The listing builds one solid part. Answer for the finished solid, in the listing's coordinates (mm). Face numbers are marked on the shaded views. A direction names the side the tool comes from. Round coordinates to 2 decimals unless told otherwise and drop trailing zeros. Loops run counter-clockwise (first coordinate to the right, second up) from the corner with the lowest first, then second, coordinate; pieces in that order, holes last. Notation, with made-up numbers: M 9,-17 L 44,-17 A31 ccw 44,9 Z; hole C -31.75,-27 d10. An arc over 180 degrees is marked long. Put each result on its own line as item: value. Start each with the question number.
(1) Straight lines are drawn through the part: line 1 (X direction, y = 12, z = 17.5); line 2 (X direction, y = 63, z = 2.25); line 3 (Z direction, x = 52, y = 34). For each, find the intervals that lie inside material, in ascending order.
(2) Determine the mould class of the marked faces 4, 5 and 6 for opening direction X: released by +X, released by -X, zero draft, split by the parting line, or undercut.
(3) Section A-A, the plane z = 22 is taken. Determine the outline of the cut face in (x, y).
(4) Section C-C, the plane x = 10 is taken. Determine the outline of the cut face in (y, z), then the cut area to 3 significant figures.
(5) Section B-B, the plane y = 14.5 is taken. Determine the outline of the cut face in (x, z), then the cut area to 3 significant figures.
(6) Flat-ended cylindrical pins translate along their axes: P1, Ø10, axis at x = 51, y = 19.5, coming from the -Z side; P2, Ø10.5, axis at y = 41.5, z = 10.5, coming from the +X side; P3, Ø21, axis at x = 71.5, y = 27, coming from the +Z side; P4, Ø6.5, axis at y = 34, z = 11.5, coming from the -X side. Find the tip coordinate at first contact, or state that the pin passes through.
(7) Which of the six approach directions +Z, -Z, +X, -X, +Y, -Y give full straight-line access (tool end or side, diameter ignored) to the marked faces 1, 2 and 3?
(8) Section D-D, the plane z = 2.75 is taken. Determine the outline of the cut face in (x, y), then the cut area to 3 significant figures.
```python
from build123d import *

# Parameters (mm, degrees)
SKETCH_1_W          = 120
SKETCH_1_H          = 75
EXTRUDE_1_DEPTH     = 4
SKETCH_2_W          = 5
SKETCH_2_H          = 75
EXTRUDE_2_DEPTH     = 21
CUT_EXTRUDE_1_DEPTH = 144.701078632


with BuildPart() as part:
    # 草图1 → 凸台-拉伸1 (new body)
    with BuildSketch(Plane.XY):
        with Locations((60, 37.5)):
            Rectangle(SKETCH_1_W, SKETCH_1_H)
    extrude(amount=EXTRUDE_1_DEPTH)

    # 草图2 → 凸台-拉伸2 (add)
    with BuildSketch(Plane.XY.offset(4)):
        with Locations((22.5, 37.5)):
            Rectangle(SKETCH_2_W, SKETCH_2_H)
        with Locations((97.5, 37.5)):
            Rectangle(SKETCH_2_W, SKETCH_2_H)
    extrude(amount=EXTRUDE_2_DEPTH)

    # 草图3 → 切除-拉伸1 (cut, through all)
    with BuildSketch(Plane(origin=(0, 0, 0), x_dir=(-1, 0, 0), z_dir=(0, 0, -1))):
        with BuildLine():
            Line((-112.5, 65), (-112.5, 55))
            ThreePointArc((-112.5, 55), (-110, 52.5), (-107.5, 55))
            Line((-107.5, 55), (-107.5, 65))
            ThreePointArc((-107.5, 65), (-110, 67.5), (-112.5, 65))
        make_face()
        with BuildLine():
            Line((-107.5, 10), (-107.5, 20))
            ThreePointArc((-107.5, 20), (-110, 22.5), (-112.5, 20))
            Line((-112.5, 20), (-112.5, 10))
            ThreePointArc((-112.5, 10), (-110, 7.5), (-107.5, 10))
        make_face()
        with BuildLine():
            Line((-7.5, 10), (-7.5, 20))
            ThreePointArc((-7.5, 20), (-10, 22.5), (-12.5, 20))
            Line((-12.5, 20), (-12.5, 10))
            ThreePointArc((-12.5, 10), (-10, 7.5), (-7.5, 10))
        make_face()
        with BuildLine():
            Line((-12.5, 65), (-12.5, 55))
            ThreePointArc((-12.5, 55), (-10, 52.5), (-7.5, 55))
            Line((-7.5, 55), (-7.5, 65))
            ThreePointArc((-7.5, 65), (-10, 67.5), (-12.5, 65))
        make_face()
    extrude(amount=-CUT_EXTRUDE_1_DEPTH, mode=Mode.SUBTRACT)


solid = part.part
```
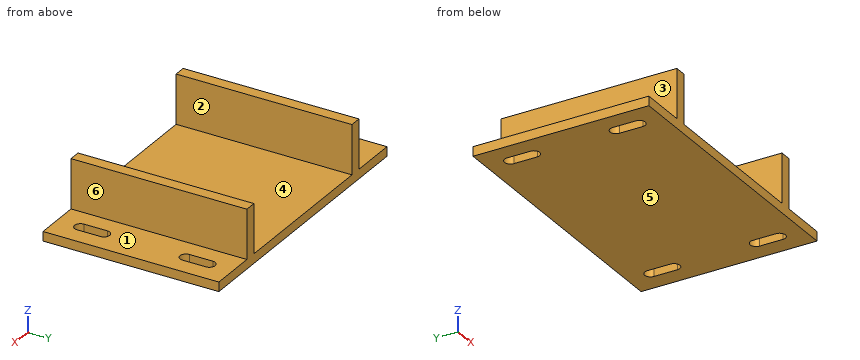
Recorded:
1. line 1: x = 20 to 25, 95 to 100
1. line 2: x = 0 to 7.5, 12.5 to 107.5, 112.5 to 120
1. line 3: z = 0 to 4
2. face 4: undercut
2. face 5: zero draft
2. face 6: released by +X
3. outline: M 20,0 L 25,0 L 25,75 L 20,75 Z; M 95,0 L 100,0 L 100,75 L 95,75 Z
4. outline: M 0,0 L 7.5,0 L 7.5,4 L 0,4 Z; M 22.5,0 L 52.5,0 L 52.5,4 L 22.5,4 Z; M 67.5,0 L 75,0 L 75,4 L 67.5,4 Z
4. area: 180 mm²
5. outline: M 0,0 L 7.5,0 L 7.5,4 L 0,4 Z; M 12.5,0 L 107.5,0 L 107.5,4 L 100,4 L 100,25 L 95,25 L 95,4 L 25,4 L 25,25 L 20,25 L 20,4 L 12.5,4 Z; M 112.5,0 L 120,0 L 120,4 L 112.5,4 Z
5. area: 650 mm²
6. P1: stops at z = 0
6. P2: stops at x = 100
6. P3: stops at z = 4
6. P4: stops at x = 20
7. face 1: +Z, +X, +Y, -Y
7. face 2: +Z, +Y, -Y
7. face 3: +Z, -X, +Y, -Y
8. outline: M 0,0 L 120,0 L 120,75 L 0,75 Z; hole M 7.5,10 A2.5 ccw 12.5,10 L 12.5,20 A2.5 ccw 7.5,20 Z; hole M 7.5,55 A2.5 ccw 12.5,55 L 12.5,65 A2.5 ccw 7.5,65 Z; hole M 107.5,10 A2.5 ccw 112.5,10 L 112.5,20 A2.5 ccw 107.5,20 Z; hole M 107.5,55 A2.5 ccw 112.5,55 L 112.5,65 A2.5 ccw 107.5,65 Z
8. area: 8,720 mm²
